CAD build for the part. Positions are in the model's coordinates, mm. A direction names the side the tool comes from. Coordinates: 2 decimals unless noted, no trailing zeros. Loops run counter-clockwise (first coordinate to the right, second up) from the corner with the lowest first, then second, coordinate; pieces in that order, holes last. Notation, with made-up numbers: (58, -26.75) - (104, -26.75) arc R3 ccw to (104, -21.75) - close; hole circle Ø10 at (84, 81). An arc over 180 degrees is marked (long way). Put each result on its own line as item: value.
```python
from build123d import *

# Parameters (mm, degrees)
F1_DEPTH = 3
F3_DEPTH = 5
F4_R     = 2.5
F5_DEPTH = 3.001


with BuildPart() as f1:
    # F0 (on Top) → F1 (new body)
    with BuildSketch(Plane.XY):
        with BuildLine():
            Line((43, -35), (43, 35))
            Line((43, 35), (32.765264, 35))
            ThreePointArc((32.765264, 35), (-4.63935, 56.943367), (-35.022314, 26))
            Line((-35.022314, 26), (-50, 26))
            Line((-50, 26), (-50, -26))
            Line((-50, -26), (-35.022314, -26))
            ThreePointArc((-35.022314, -26), (-4.63935, -56.943367), (32.765264, -35))
            Line((32.765264, -35), (43, -35))
        make_face()
    extrude(amount=F1_DEPTH)

    # F2 (on face) → F3 (join)
    with BuildSketch(Plane.XY.offset(3)):
        with BuildLine():
            Line((-34.799137, 8.656902), (-30.455283, 8.656902))
            ThreePointArc((-30.455283, 8.656902), (-9.079543, 53.986316), (32.923604, 26.647449))
            Line((32.923604, 26.647449), (43, 28.911306))
            Line((43, 28.911306), (43, 35))
            Line((43, 35), (32.765264, 35))
            ThreePointArc((32.765264, 35), (-4.63935, 56.943367), (-35.022314, 26))
            Line((-35.022314, 26), (-50, 26))
            Line((-50, 26), (-50, 17.479896))
            Line((-50, 17.479896), (-34.799137, 8.656902))
        make_face()
        with BuildLine():
            Line((43, -28.911306), (32.923604, -26.647449))
            ThreePointArc((32.923604, -26.647449), (-9.079543, -53.986316), (-30.455283, -8.656902))
            Line((-30.455283, -8.656902), (-34.799137, -8.656902))
            Line((-34.799137, -8.656902), (-50, -17.479896))
            Line((-50, -17.479896), (-50, -26))
            Line((-50, -26), (-35.022314, -26))
            ThreePointArc((-35.022314, -26), (-4.63935, -56.943367), (32.765264, -35))
            Line((32.765264, -35), (43, -35))
            Line((43, -35), (43, -28.911306))
        make_face()
        with BuildLine():
            Line((43, 16.62755), (32.329441, 14.230203))
            ThreePointArc((32.329441, 14.230203), (31.476652, 11.286323), (30.356414, 8.433473))
            Line((30.356414, 8.433473), (43, 8.433473))
            Line((43, 8.433473), (43, 16.62755))
        make_face()
        with BuildLine():
            Line((43, -8.433473), (30.356414, -8.433473))
            ThreePointArc((30.356414, -8.433473), (31.476652, -11.286323), (32.329441, -14.230203))
            Line((32.329441, -14.230203), (43, -16.62755))
            Line((43, -16.62755), (43, -8.433473))
        make_face()
    extrude(amount=F3_DEPTH)

    # F4 (on face) → F5 (cut, through all)
    with BuildSketch(Plane.XY.offset(3)):
        with Locations((0, 22)):
            Circle(F4_R)
        with Locations((0, -22)):
            Circle(F4_R)
    extrude(amount=-F5_DEPTH, mode=Mode.SUBTRACT)


solid = f1.part
```
Q1. Slice it at D-D, the plane x = -23. Give the cut face in (y, z), then the cut area to 3 significant figures.
Determined:
outline: (-48.71, 0) - (48.71, 0) - (48.71, 8) - (46.01, 8) - (46.01, 3) - (-46.01, 3) - (-46.01, 8) - (-48.71, 8) - close
area: 319 mm2
Q2. Slice it at A-A, the plane z = 6. Give the cut face in (x, y).
Determined:
outline: (-50, -26) - (-35.02, -26) arc R35.25 ccw to (32.77, -35) - (43, -35) - (43, -28.91) - (32.92, -26.65) arc R33.25 cw (long way) to (-30.46, -8.66) - (-34.8, -8.66) - (-50, -17.48) - close; (-50, 17.48) - (-34.8, 8.66) - (-30.46, 8.66) arc R33.25 cw (long way) to (32.92, 26.65) - (43, 28.91) - (43, 35) - (32.77, 35) arc R35.25 ccw to (-35.02, 26) - (-50, 26) - close; (30.36, -8.43) arc R33.25 cw to (32.33, -14.23) - (43, -16.63) - (43, -8.43) - close; (30.36, 8.43) - (43, 8.43) - (43, 16.63) - (32.33, 14.23) arc R33.25 cw to start
Q3. Pin check, flat tips, straight feed: pin 1 Ø8 at (x, y) = (30, -1) entering from +Z; pin 2 Ø1.5 at (x, z) = (-12, 4.5) entering from -Y; pin 3 Ø1.5 at (x, z) = (35, 4.5) entering from +Y. Stop position of each tip, or through.
Determined:
pin 1: z = 3
pin 2: y = -55.41
pin 3: y = 35
Q4. Mould opens along X. For faces 6 (the cylindrical face through (-3.99, 57.023, 3.944)), 7 (the cylindrical face through (31.463, -11.246, 5.465)), 8 (the flat face through (38, 12, 8)), 9 (the cylindrical face through (-8.313, -54.194, 5.465)) say: +X half, -X half, draft (parallel to the pull), parting line (faces both ways), or undercut.
Determined:
face 6: parting line
face 7: undercut
face 8: draft
face 9: undercut
Q5. Wall check: L1, parallel to Y at x = 0, z = 2.25; L2, parallel to Y at x = 0, z = 6.5; L3, parallel to X at y = 37.5, z = 6. Give the ranges that are in metal, low to high. Write a range as from..to.
Determined:
L1: -57.25..-24.5, -19.5..19.5, 24.5..57.25
L2: -57.25..-55.25, 55.25..57.25
L3: -31.66..-29.42, 29.42..31.66
Q6. Tool access for faces 1 (the cylindrical face through (31.49, 11.33, 5.46)), 2 (the flat face through (37, 8.433, 5)), 3 (the flat face through (-33, -8.657, 5)), 4 (the flat face through (-42, 26, 4)), 5 (the flat face through (37.891, 27.764, 5.465)): list every direction of +Z, -Z, +X, -X, +Y, -Y with a clear straight run to the whole face (end or side of a thin tool).
Determined:
face 1: +Z
face 2: +Z, +X, -X
face 3: +Z, -X
face 4: +Z, -Z, -X, +Y
face 5: +Z, +X
Q7. Slice it at C-C, the plane y = 22. Give the cut face in (x, z).
Determined:
outline: (-50, 0) - (-2.5, 0) - (-2.5, 3) - (-33.25, 3) - (-33.25, 8) - (-50, 8) - close; (2.5, 0) - (43, 0) - (43, 3) - (2.5, 3) - close
Q8. Slice it at B-B, the plane x = 0. Give the cut face in (y, z), then the cut area to 4 significant figures.
Determined:
outline: (-57.25, 0) - (-24.5, 0) - (-24.5, 3) - (-55.25, 3) - (-55.25, 8) - (-57.25, 8) - close; (-19.5, 0) - (19.5, 0) - (19.5, 3) - (-19.5, 3) - close; (24.5, 0) - (57.25, 0) - (57.25, 8) - (55.25, 8) - (55.25, 3) - (24.5, 3) - close
area: 333.5 mm2
